Build history of the part. All positions in model axes, mm. Face numbers are marked on the shaded views. A direction names the side the tool comes from. Coordinates: 2 decimals unless noted, no trailing zeros. Order: outer loops, then holes, each group sorted by start corner. A loop starts at its lowest first (then second) coordinate and runs counter-clockwise, first axis right, second up. Notation, with made-up numbers: M 82,22 L 96,22 A26 ccw 96,48 Z; hole C -1,20.5 d5. An arc over 180 degrees is marked long. Use a Markdown table: item, result. Add a question column.
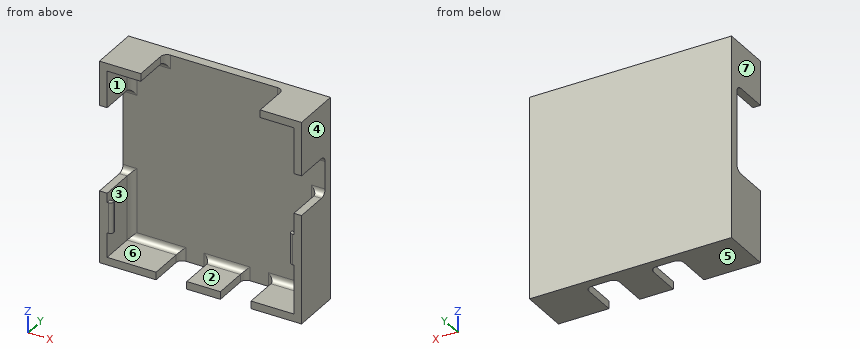
from build123d import *

# Parameters (mm, degrees)
SKETCH1_W           = 66
SKETCH1_H           = 66
BOSS_EXTRUDE1_DEPTH = 3
SKETCH2_W           = 11
SKETCH2_H           = 2.5
BOSS_EXTRUDE3_DEPTH = 13
SKETCH5_W           = 10
SKETCH5_H           = 1.5
BOSS_EXTRUDE4_DEPTH = 1.5
FILLET2_R           = 1
SKETCH6_W           = 10
SKETCH6_H           = 1.5
BOSS_EXTRUDE5_DEPTH = 1.5
FILLET3_R           = 1
FILLET4_R           = 2


with BuildPart() as part:
    # Sketch1 → Boss-Extrude1 (new body)
    with BuildSketch(Plane(origin=(0, 0, 0), x_dir=(1, 0, 0), z_dir=(0, 1, 0))):
        Rectangle(SKETCH1_W, SKETCH1_H)
    extrude(amount=BOSS_EXTRUDE1_DEPTH)

    # Sketch2 → Boss-Extrude3 (add)
    with BuildSketch(Plane(origin=(0, 0, 0), x_dir=(1, 0, 0), z_dir=(0, 1, 0))):
        Polygon((-30.5, 30.5), (-14.5, 30.5), (-14.5, 33), (-33, 33), (-33, 9.5), (-30.5, 9.5), align=None)
        Polygon((-30.5, -30.5), (-19.5, -30.5), (-19.5, -33), (-33, -33), (-33, -18.5), (-30.5, -18.5), align=None)
        Polygon((30.5, 30.5), (30.5, -2.5), (33, -2.5), (33, 33), (16.5, 33), (16.5, 30.5), align=None)
        with Locations((1, 31.75)):
            Rectangle(SKETCH2_W, SKETCH2_H)
        Polygon((30.5, -15.5), (33, -15.5), (33, -33), (19.5, -33), (19.5, -30.5), (30.5, -30.5), align=None)
    extrude(amount=-BOSS_EXTRUDE3_DEPTH)

    # Sketch5 → Boss-Extrude4 (add)
    with BuildSketch(Plane.ZY.offset(-30.5)):
        with Locations((-9.5, -12.25)):
            Rectangle(SKETCH5_W, SKETCH5_H)
    extrude(amount=BOSS_EXTRUDE4_DEPTH)

    # Fillet2
    fillet2_edges = [part.edges().sort_by_distance(p)[0] for p in [
        (29, -13, -9.5),
    ]]
    fillet(fillet2_edges, radius=FILLET2_R)

    # Sketch6 → Boss-Extrude5 (add)
    with BuildSketch(Plane(origin=(-30.5, 0, 0), x_dir=(0, 0, -1), z_dir=(1, 0, 0))):
        with Locations((17.5, -12.25)):
            Rectangle(SKETCH6_W, SKETCH6_H)
    extrude(amount=BOSS_EXTRUDE5_DEPTH)

    # Fillet3
    fillet3_edges = [part.edges().sort_by_distance(p)[0] for p in [
        (-29, -13, -17.5),
    ]]
    fillet(fillet3_edges, radius=FILLET3_R)

    # Fillet4
    fillet4_edges = [part.edges().sort_by_distance(p)[0] for p in [
        (31.75, 0, 15.5),
        (-31.75, 0, 18.5),
        (19.5, 0, 31.75),
        (-4.5, 0, -31.75),
        (31.75, 0, 2.5),
        (-19.5, 0, 31.75),
        (-31.75, 0, -9.5),
        (-14.5, 0, -31.75),
        (6.5, 0, -31.75),
        (16.5, 0, -31.75),
        (25, 0, 30.5),
        (-25, 0, 30.5),
        (-30.5, 0, 24.5),
        (30.5, 0, 23),
        (30.5, 0, -14),
        (23.5, 0, -30.5),
        (1, 0, -30.5),
        (-22.5, 0, -30.5),
        (-30.5, 0, -20),
    ]]
    fillet(fillet4_edges, radius=FILLET4_R)


solid = part.part
(1) Mould opens along X. For the marked faces 5, 6 and 7 say: released by +X, released by -X, zero draft, split by the parting line, or undercut.
(2) Which spindle directions (+Z, -Z, +X, -X, +Y, -Y) get a long thin tool onto all of the face, cutting with end or side? Do the marked faces 1, 2, 3 and 4. Say none if no direction does.
(3) Slice it at B-B on y = -3. Give the cut face in (x, z), and give its area (3 significant figures).
(4) Slice it at D-D on x = 25. Give the cut face in (y, z).
(5) Slice it at A-A on x = -1. Give the cut face in (y, z), and give its area (3 significant figures).
(6) Slice it at C-C on z = -3. Give the cut face in (x, y), and give its area (3 significant figures).
(7) Drill centre lines: line 1 along Z through (x, y) = (26.5, -11.75); line 2 along Y through (x, z) = (-16, -21). Where is each one in solid material? Low to high. Write a range as from..to.
(8) Drop flat-ended pins along their axis: P1, Ø2, axis at x = 24, z = -12.5, coming from the -Y side; P2, Ø3.5, axis at y = -5.5, z = -7, coming from the -X side; P3, Ø5.5, axis at x = 1, y = -8, coming from the +Z side. Give the stop position or say it passes through.
Solutions:
| question | item | result |
|---|---|---|
| 1 | face 5 | zero draft |
| 1 | face 6 | undercut |
| 1 | face 7 | released by -X |
| 2 | face 1 | -Y |
| 2 | face 2 | +Z, -Y |
| 2 | face 3 | none |
| 2 | face 4 | +Z, -Z, +X, +Y, -Y |
| 3 | outline | M -33,-33 L -14.5,-33 L -14.5,-30.5 L -30.5,-30.5 L -30.5,-9.5 L -33,-9.5 Z; M -33,18.5 L -30.5,18.5 L -30.5,30.5 L -19.5,30.5 L -19.5,33 L -33,33 Z; M -4.5,-33 L 6.5,-33 L 6.5,-30.5 L -4.5,-30.5 Z; M 16.5,-33 L 33,-33 L 33,2.5 L 30.5,2.5 L 30.5,-30.5 L 16.5,-30.5 Z; M 19.5,30.5 L 30.5,30.5 L 30.5,15.5 L 33,15.5 L 33,33 L 19.5,33 Z |
| 3 | area | 385 mm² |
| 4 | outline | M -13,-33 L 3,-33 L 3,33 L -13,33 L -13,30.5 L -2,30.5 A2 cw 0,28.5 L 0,-28.5 A2 cw -2,-30.5 L -13,-30.5 Z |
| 5 | outline | M -13,-33 L 3,-33 L 3,33 L 0,33 L 0,-28.5 A2 cw -2,-30.5 L -13,-30.5 Z |
| 5 | area | 231 mm² |
| 6 | outline | M -33,0 L 28.5,0 A2 cw 30.5,-2 L 30.5,-13 L 33,-13 L 33,3 L -33,3 Z |
| 6 | area | 231 mm² |
| 7 | line 1 | -33..-30.5, 30.5..33 |
| 7 | line 2 | 0..3 |
| 8 | P1 | y = 0 |
| 8 | P2 | x = 30.5 |
| 8 | P3 | z = -30.5 |
